Geometry: final body of the model. Coordinates: model frame, mm. Give positions to 0.01 mm unless a question says otherwise; leave off trailing zeros. Write each loop counter-clockwise with the first axis right and the second up, starting at its lowest first coordinate (ties: lowest second). Pieces come first, ordered by that corner, then holes.
from build123d import *

# Parameters (mm, degrees)
SKETCH1_W                = 400
SKETCH1_H                = 360
BOSS_EXTRUDE1_DEPTH      = 4
SKETCH2_W                = 100
SKETCH2_H                = 55
CORNER_DEPTH             = 4
SKETCH3_R                = 2.25
MOTOR_MOUNTING_DEPTH     = 4
MIRROR2_COPY_1_SKETCH_W  = 100
MIRROR2_COPY_1_SKETCH_H  = 55
MIRROR2_COPY_1_DEPTH     = 4
MIRROR2_COPY_2_SKETCH_R  = 2.25
MIRROR2_COPY_2_DEPTH     = 4
PC_MOUNTING_REACH        = 6
SKETCH5_R                = 1.5
ARDUINO_MOUNTING_REACH   = 6
SKETCH6_R                = 1.25
DCDC_USB_MOUNTING_REACH  = 6
SKETCH7_R                = 2
SKETCH10_W               = 20
SKETCH10_H               = 4
SKETCH10_W_2             = 4
SKETCH10_H_2             = 24
SKETCH10_W_3             = 5
SKETCH10_W_4             = 7.47
SIDES_MOUNTING_DEPTH     = 5
SKETCH11_W               = 30
SKETCH11_H               = 4
SKETCH11_W_2             = 25
FIN_MOUNTING_DEPTH       = 5
M4_CLEARANCE_HOLE1_D     = 4.3
M4_CLEARANCE_HOLE1_DEPTH = 6
M4_CLEARANCE_HOLE1_TIP   = 1.291850331
M6_CLEARANCE_HOLE1_D     = 6.4
M6_CLEARANCE_HOLE1_DEPTH = 6
M6_CLEARANCE_HOLE1_TIP   = 1.922753981


with BuildPart() as part:
    # Sketch1 → Boss-Extrude1 (new body)
    with BuildSketch(Plane(origin=(0, 0, 0), x_dir=(1, 0, 0), z_dir=(0, 1, 0))):
        Rectangle(SKETCH1_W, SKETCH1_H)
    extrude(amount=BOSS_EXTRUDE1_DEPTH)

    # Sketch2 → Corner (cut)
    with BuildSketch(Plane(origin=(0, 4, 0), x_dir=(1, 0, 0), z_dir=(0, 1, 0))):
        with Locations((-150, 152.5)):
            Rectangle(SKETCH2_W, SKETCH2_H)
    corner = extrude(amount=-CORNER_DEPTH, mode=Mode.SUBTRACT)

    # Sketch3 → Motor mounting (cut)
    with BuildSketch(Plane(origin=(0, 4, 0), x_dir=(1, 0, 0), z_dir=(0, 1, 0))):
        with Locations((-179.05, 112.5)):
            Circle(SKETCH3_R)
        with Locations((-128.25, 112.5)):
            Circle(SKETCH3_R)
        with Locations((-160, 99.8)):
            Circle(SKETCH3_R)
    motor_mounting = extrude(amount=-MOTOR_MOUNTING_DEPTH, mode=Mode.SUBTRACT)

    # Mirror1: Corner, Motor mounting across plane
    add(corner.mirror(Plane.XY), mode=Mode.SUBTRACT)
    add(motor_mounting.mirror(Plane.XY), mode=Mode.SUBTRACT)

    # Mirror2: Corner, Motor mounting across plane
    add(corner.mirror(Plane(origin=(0, 0, 0), x_dir=(0, 0, 1), z_dir=(1, 0, 0))), mode=Mode.SUBTRACT)
    add(motor_mounting.mirror(Plane(origin=(0, 0, 0), x_dir=(0, 0, 1), z_dir=(1, 0, 0))), mode=Mode.SUBTRACT)

    # Mirror2 copy 1 sketch → Mirror2 copy 1 (cut)
    with BuildSketch(Plane(origin=(0, 4, 0), x_dir=(-1, 0, 0), z_dir=(0, 1, 0))):
        with Locations((-150, 152.5)):
            Rectangle(MIRROR2_COPY_1_SKETCH_W, MIRROR2_COPY_1_SKETCH_H)
    extrude(amount=-MIRROR2_COPY_1_DEPTH, mode=Mode.SUBTRACT)

    # Mirror2 copy 2 sketch → Mirror2 copy 2 (cut)
    with BuildSketch(Plane(origin=(0, 4, 0), x_dir=(-1, 0, 0), z_dir=(0, 1, 0))):
        with Locations((-179.05, 112.5)):
            Circle(MIRROR2_COPY_2_SKETCH_R)
        with Locations((-128.25, 112.5)):
            Circle(MIRROR2_COPY_2_SKETCH_R)
        with Locations((-160, 99.8)):
            Circle(MIRROR2_COPY_2_SKETCH_R)
    extrude(amount=-MIRROR2_COPY_2_DEPTH, mode=Mode.SUBTRACT)

    # Sketch5 → PC mounting (cut, up to next)
    with BuildSketch(Plane(origin=(0, 4, 0), x_dir=(1, 0, 0), z_dir=(0, 1, 0)), mode=Mode.PRIVATE) as pc_mounting_sk1:
        with Locations((-78.74, 156.73)):
            Circle(SKETCH5_R)
    pc_mounting_tool1 = extrude(pc_mounting_sk1.sketch, amount=-PC_MOUNTING_REACH, mode=Mode.PRIVATE) & part.part
    add(pc_mounting_tool1.solids().sort_by_distance((-78.74, 4, -156.73))[0], mode=Mode.SUBTRACT)
    # Sketch5 → PC mounting (cut, up to next)
    with BuildSketch(Plane(origin=(0, 4, 0), x_dir=(1, 0, 0), z_dir=(0, 1, 0)), mode=Mode.PRIVATE) as pc_mounting_sk2:
        with Locations((78.74, 133.87)):
            Circle(SKETCH5_R)
    pc_mounting_tool2 = extrude(pc_mounting_sk2.sketch, amount=-PC_MOUNTING_REACH, mode=Mode.PRIVATE) & part.part
    add(pc_mounting_tool2.solids().sort_by_distance((78.74, 4, -133.87))[0], mode=Mode.SUBTRACT)
    # Sketch5 → PC mounting (cut, up to next)
    with BuildSketch(Plane(origin=(0, 4, 0), x_dir=(1, 0, 0), z_dir=(0, 1, 0)), mode=Mode.PRIVATE) as pc_mounting_sk3:
        with Locations((-78.74, 1.79)):
            Circle(SKETCH5_R)
    pc_mounting_tool3 = extrude(pc_mounting_sk3.sketch, amount=-PC_MOUNTING_REACH, mode=Mode.PRIVATE) & part.part
    add(pc_mounting_tool3.solids().sort_by_distance((-78.74, 4, -1.79))[0], mode=Mode.SUBTRACT)
    # Sketch5 → PC mounting (cut, up to next)
    with BuildSketch(Plane(origin=(0, 4, 0), x_dir=(1, 0, 0), z_dir=(0, 1, 0)), mode=Mode.PRIVATE) as pc_mounting_sk4:
        with Locations((78.74, 1.79)):
            Circle(SKETCH5_R)
    pc_mounting_tool4 = extrude(pc_mounting_sk4.sketch, amount=-PC_MOUNTING_REACH, mode=Mode.PRIVATE) & part.part
    add(pc_mounting_tool4.solids().sort_by_distance((78.74, 4, -1.79))[0], mode=Mode.SUBTRACT)

    # Sketch6 → Arduino mounting (cut, up to next)
    with BuildSketch(Plane(origin=(0, 4, 0), x_dir=(1, 0, 0), z_dir=(0, 1, 0)), mode=Mode.PRIVATE) as arduino_mounting_sk1:
        with Locations((56.8, -37.9)):
            Circle(SKETCH6_R)
    arduino_mounting_tool1 = extrude(arduino_mounting_sk1.sketch, amount=-ARDUINO_MOUNTING_REACH, mode=Mode.PRIVATE) & part.part
    add(arduino_mounting_tool1.solids().sort_by_distance((56.8, 4, 37.9))[0], mode=Mode.SUBTRACT)
    # Sketch6 → Arduino mounting (cut, up to next)
    with BuildSketch(Plane(origin=(0, 4, 0), x_dir=(1, 0, 0), z_dir=(0, 1, 0)), mode=Mode.PRIVATE) as arduino_mounting_sk2:
        with Locations((105, -39.2)):
            Circle(SKETCH6_R)
    arduino_mounting_tool2 = extrude(arduino_mounting_sk2.sketch, amount=-ARDUINO_MOUNTING_REACH, mode=Mode.PRIVATE) & part.part
    add(arduino_mounting_tool2.solids().sort_by_distance((105, 4, 39.2))[0], mode=Mode.SUBTRACT)
    # Sketch6 → Arduino mounting (cut, up to next)
    with BuildSketch(Plane(origin=(0, 4, 0), x_dir=(1, 0, 0), z_dir=(0, 1, 0)), mode=Mode.PRIVATE) as arduino_mounting_sk3:
        with Locations((89.8, -90)):
            Circle(SKETCH6_R)
    arduino_mounting_tool3 = extrude(arduino_mounting_sk3.sketch, amount=-ARDUINO_MOUNTING_REACH, mode=Mode.PRIVATE) & part.part
    add(arduino_mounting_tool3.solids().sort_by_distance((89.8, 4, 90))[0], mode=Mode.SUBTRACT)
    # Sketch6 → Arduino mounting (cut, up to next)
    with BuildSketch(Plane(origin=(0, 4, 0), x_dir=(1, 0, 0), z_dir=(0, 1, 0)), mode=Mode.PRIVATE) as arduino_mounting_sk4:
        with Locations((61.9, -90)):
            Circle(SKETCH6_R)
    arduino_mounting_tool4 = extrude(arduino_mounting_sk4.sketch, amount=-ARDUINO_MOUNTING_REACH, mode=Mode.PRIVATE) & part.part
    add(arduino_mounting_tool4.solids().sort_by_distance((61.9, 4, 90))[0], mode=Mode.SUBTRACT)

    # Sketch7 → DCDC-USB mounting (cut, up to next)
    with BuildSketch(Plane(origin=(0, 4, 0), x_dir=(1, 0, 0), z_dir=(0, 1, 0)), mode=Mode.PRIVATE) as dcdc_usb_mounting_sk1:
        with Locations((-115, -75)):
            Circle(SKETCH7_R)
    dcdc_usb_mounting_tool1 = extrude(dcdc_usb_mounting_sk1.sketch, amount=-DCDC_USB_MOUNTING_REACH, mode=Mode.PRIVATE) & part.part
    add(dcdc_usb_mounting_tool1.solids().sort_by_distance((-115, 4, 75))[0], mode=Mode.SUBTRACT)
    # Sketch7 → DCDC-USB mounting (cut, up to next)
    with BuildSketch(Plane(origin=(0, 4, 0), x_dir=(1, 0, 0), z_dir=(0, 1, 0)), mode=Mode.PRIVATE) as dcdc_usb_mounting_sk2:
        with Locations((15.6, -75)):
            Circle(SKETCH7_R)
    dcdc_usb_mounting_tool2 = extrude(dcdc_usb_mounting_sk2.sketch, amount=-DCDC_USB_MOUNTING_REACH, mode=Mode.PRIVATE) & part.part
    add(dcdc_usb_mounting_tool2.solids().sort_by_distance((15.6, 4, 75))[0], mode=Mode.SUBTRACT)
    # Sketch7 → DCDC-USB mounting (cut, up to next)
    with BuildSketch(Plane(origin=(0, 4, 0), x_dir=(1, 0, 0), z_dir=(0, 1, 0)), mode=Mode.PRIVATE) as dcdc_usb_mounting_sk3:
        with Locations((-115, -23.4)):
            Circle(SKETCH7_R)
    dcdc_usb_mounting_tool3 = extrude(dcdc_usb_mounting_sk3.sketch, amount=-DCDC_USB_MOUNTING_REACH, mode=Mode.PRIVATE) & part.part
    add(dcdc_usb_mounting_tool3.solids().sort_by_distance((-115, 4, 23.4))[0], mode=Mode.SUBTRACT)
    # Sketch7 → DCDC-USB mounting (cut, up to next)
    with BuildSketch(Plane(origin=(0, 4, 0), x_dir=(1, 0, 0), z_dir=(0, 1, 0)), mode=Mode.PRIVATE) as dcdc_usb_mounting_sk4:
        with Locations((15.6, -23.4)):
            Circle(SKETCH7_R)
    dcdc_usb_mounting_tool4 = extrude(dcdc_usb_mounting_sk4.sketch, amount=-DCDC_USB_MOUNTING_REACH, mode=Mode.PRIVATE) & part.part
    add(dcdc_usb_mounting_tool4.solids().sort_by_distance((15.6, 4, 23.4))[0], mode=Mode.SUBTRACT)

    # Sketch10 → Sides mounting (cut, through all)
    with BuildSketch(Plane(origin=(0, 4, 0), x_dir=(1, 0, 0), z_dir=(0, 1, 0))):
        with Locations((-68, 171)):
            Rectangle(SKETCH10_W, SKETCH10_H)
        with Locations((-191, 78)):
            Rectangle(SKETCH10_W_2, SKETCH10_H_2)
        with Locations((-191, -42)):
            Rectangle(SKETCH10_W_2, SKETCH10_H_2)
        with Locations((-191, -78)):
            Rectangle(SKETCH10_W_2, SKETCH10_H_2)
        with Locations((-191, 42)):
            Rectangle(SKETCH10_W_2, SKETCH10_H_2)
        with Locations((191, 78)):
            Rectangle(SKETCH10_W_2, SKETCH10_H_2)
        with Locations((191, 42)):
            Rectangle(SKETCH10_W_2, SKETCH10_H_2)
        with Locations((191, -42)):
            Rectangle(SKETCH10_W_2, SKETCH10_H_2)
        with Locations((191, -78)):
            Rectangle(SKETCH10_W_2, SKETCH10_H_2)
        with Locations((-65, -171)):
            Rectangle(SKETCH10_W, SKETCH10_H)
        with Locations((-33, -171)):
            Rectangle(SKETCH10_W, SKETCH10_H)
        with Locations((33, -171)):
            Rectangle(SKETCH10_W, SKETCH10_H)
        with Locations((65, -171)):
            Rectangle(SKETCH10_W, SKETCH10_H)
        with Locations((-92.5, 171)):
            Rectangle(SKETCH10_W_3, SKETCH10_H)
        with Locations((91.265, 171)):
            Rectangle(SKETCH10_W_4, SKETCH10_H)
    extrude(amount=-SIDES_MOUNTING_DEPTH, mode=Mode.SUBTRACT)

    # Sketch11 → fin mounting (cut, through all)
    with BuildSketch(Plane(origin=(0, 4, 0), x_dir=(1, 0, 0), z_dir=(0, 1, 0))):
        with Locations((154, 8.5)):
            Rectangle(SKETCH11_W, SKETCH11_H)
        with Locations((114.5, 8.5)):
            Rectangle(SKETCH11_W_2, SKETCH11_H)
        with Locations((114.5, -8.5)):
            Rectangle(SKETCH11_W_2, SKETCH11_H)
        with Locations((154, -8.5)):
            Rectangle(SKETCH11_W, SKETCH11_H)
    extrude(amount=-FIN_MOUNTING_DEPTH, mode=Mode.SUBTRACT)

    # M4 Clearance Hole1
    with Locations(Plane(origin=(0, 4, 0), x_dir=(-1, 0, 0), z_dir=(0, 1, 0))):
        with Locations((49, 171), (-49, 171), (191, 60), (191, -60), (-133, -8.5), (-191, -60), (-191, 60), (84, -171), (-133, 8.5)):
            Hole(M4_CLEARANCE_HOLE1_D / 2, depth=M4_CLEARANCE_HOLE1_DEPTH)
            with Locations((0, 0, -(M4_CLEARANCE_HOLE1_DEPTH + M4_CLEARANCE_HOLE1_TIP / 2))):  # 118° drill point
                Cone(0, M4_CLEARANCE_HOLE1_D / 2, M4_CLEARANCE_HOLE1_TIP, mode=Mode.SUBTRACT)

    # M6 Clearance Hole1
    with Locations(Plane(origin=(0, 4, 0), x_dir=(-1, 0, 0), z_dir=(0, 1, 0))):
        with Locations((180, 0), (120, 0)):
            Hole(M6_CLEARANCE_HOLE1_D / 2, depth=M6_CLEARANCE_HOLE1_DEPTH)
            with Locations((0, 0, -(M6_CLEARANCE_HOLE1_DEPTH + M6_CLEARANCE_HOLE1_TIP / 2))):  # 118° drill point
                Cone(0, M6_CLEARANCE_HOLE1_D / 2, M6_CLEARANCE_HOLE1_TIP, mode=Mode.SUBTRACT)


solid = part.part
Q1. Section C-C on z = -140. Output: boundary loops of the cut face in (x, y).
Filled sheet:
outline: (-100, 0) - (100, 0) - (100, 4) - (-100, 4) - close
Q2. Pin query (flat end, axial travel): P1, Ø2, axis at x = -190.5, y = 3, coming from the +Z side; P2, Ø5, axis at x = 141.5, z = 67.5, coming from the -Y side; P3, Ø2, axis at y = 2, z = 171, coming from the -X side. Return the tip coordinate at first contact, or that it passes through.
Filled sheet:
P1: stops at z = 125
P2: stops at y = 0
P3: stops at x = -100
Q3. Section A-A on z = -74. Output: boundary loops of the cut face in (x, y).
Filled sheet:
outline: (-200, 0) - (-193, 0) - (-193, 4) - (-200, 4) - close; (-189, 0) - (189, 0) - (189, 4) - (-189, 4) - close; (193, 0) - (200, 0) - (200, 4) - (193, 4) - close
Q4. Section B-B on y = 2.8. Count the separate pieces of the cut face and the enclosed holes in it, plus the area to 3 significant figures.
Filled sheet:
separate pieces: 1
enclosed holes: 54
area: 120,000 mm2
Q5. Ray query, line 1 along Z through (x, y) = (-115, 1.3); line 2 along Z through (x, y) = (179.05, 2.5); line 3 along X through (y, z) = (0.85, -48). Return the intervals inside material, ascending.
Filled sheet:
line 1: z = -125 to 21.4, 25.4 to 73, 77 to 125
line 2: z = -125 to -114.75, -110.25 to 110.25, 114.75 to 125
line 3: x = -200 to -193, -189 to 189, 193 to 200
